Part model, mm, in its own coordinate system. Face numbers are marked on the shaded views. A direction names the side the tool comes from. Give positions to 0.01 mm unless a question says otherwise; leave off trailing zeros. Order: outer loops, then holes, each group sorted by start corner. A loop starts at its lowest first (then second) coordinate and runs counter-clockwise, first axis right, second up. Notation, with made-up numbers: (63, 76.25) - (95, 76.25) arc R30 cw to (95, 99.25) - close; hole circle Ø11 at (-33.5, -25.75). An arc over 180 degrees is marked (long way). One line per item, written item: value.
```python
from build123d import *

# Parameters (mm, degrees)
BOSS_EXTRU_1_DEPTH      = 9
ESQUISSE2_R             = 1
ENL_V_MAT_EXTRU_1_DEPTH = 16.588457268


with BuildPart() as part:
    # Esquisse1 → Boss.-Extru.1 (new body)
    with BuildSketch(Plane(origin=(0, 0, 0), x_dir=(1, 0, 0), z_dir=(0, 1, 0))):
        with BuildLine():
            Line((3.968626967, 0.5), (8.986100378, 0.5))
            ThreePointArc((8.986100378, 0.5), (-9, 0), (8.986100378, -0.5))
            Line((8.986100378, -0.5), (3.968626967, -0.5))
            ThreePointArc((3.968626967, -0.5), (0, -4), (-3.968626967, -0.5))
            Line((-3.968626967, -0.5), (-5, -0.5))
            Line((-5, -0.5), (-5, 0.5))
            Line((-5, 0.5), (-3.968626967, 0.5))
            ThreePointArc((-3.968626967, 0.5), (0, 4), (3.968626967, 0.5))
        make_face()
    extrude(amount=BOSS_EXTRU_1_DEPTH)

    # Esquisse2 → Enlèv. mat.-Extru.1 (cut, through all)
    with BuildSketch(Plane(origin=(0, 9, 0), x_dir=(1, 0, 0), z_dir=(0, 1, 0))):
        with Locations(Location((0, -6.5, 0), (0, 0, 270))):
            Circle(ESQUISSE2_R)
        with Locations(Location((0, 6.5, 0), (0, 0, 270))):
            Circle(ESQUISSE2_R)
    extrude(amount=-ENL_V_MAT_EXTRU_1_DEPTH, mode=Mode.SUBTRACT)


solid = part.part
```
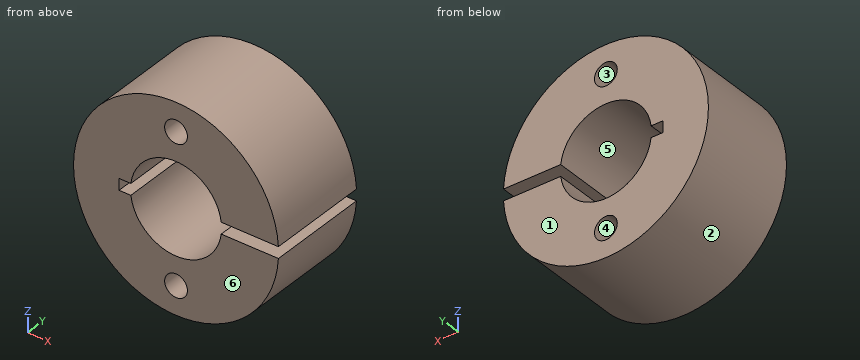
1) Cut at B-B, the plane x = 0. Give the cut face in (y, z), then the cut area to 3 significant figures.
Outcome:
outline: (0, -9) - (9, -9) - (9, -7.5) - (0, -7.5) - close; (0, -5.5) - (9, -5.5) - (9, -4) - (0, -4) - close; (0, 4) - (9, 4) - (9, 5.5) - (0, 5.5) - close; (0, 7.5) - (9, 7.5) - (9, 9) - (0, 9) - close
area: 54.0 mm^2
2) Cut at D-D, the plane x = -2.25. Give the cut face in (y, z).
Outcome:
outline: (0, -8.71) - (9, -8.71) - (9, -3.31) - (0, -3.31) - close; (0, 3.31) - (9, 3.31) - (9, 8.71) - (0, 8.71) - close
3) Drill centre lines: line 1 along X through (y, z) = (4.25, 6.5); line 2 along Z through (x, y) = (-0.25, 7.25); line 3 along Z through (x, y) = (-1.25, 7). Where is each one in solid material? Low to high. Write a range as from..to.
Outcome:
line 1: x = -6.22..-1, 1..6.22
line 2: z = -9..-7.47, -5.53..-3.99, 3.99..5.53, 7.47..9
line 3: z = -8.91..-3.8, 3.8..8.91
4) Which spindle directions (+Z, -Z, +X, -X, +Y, -Y) get a long thin tool onto all of the face, cutting with end or side? Do the marked faces 5 and 6. Say none if no direction does.
Outcome:
face 5: +Y, -Y
face 6: +Z, -Z, +X, -X, -Y
5) Mould opens along Z. For the marked faces 1, 2, 3 and 4 say: released by +Z, released by -Z, zero draft, split by the parting line, or undercut.
Outcome:
face 1: zero draft
face 2: split by the parting line
face 3: undercut
face 4: undercut
6) Cut at A-A, the plane y = 1.5. Give the cut face in (x, z), then the cut area to 3 significant figures.
Outcome:
outline: (-5, -0.5) - (-5, 0.5) - (-3.97, 0.5) arc R4 cw to (3.97, 0.5) - (8.99, 0.5) arc R9 ccw (long way) to (8.99, -0.5) - (3.97, -0.5) arc R4 cw to (-3.97, -0.5) - close; hole circle Ø2 at (0, -6.5); hole circle Ø2 at (0, 6.5)
area: 192 mm^2
7) Cut at C-C, the plane z = 3.25. Give the cut face in (x, y), then the cut area to 3 significant figures.
Outcome:
outline: (-8.39, 0) - (-2.33, 0) - (-2.33, 9) - (-8.39, 9) - close; (2.33, 0) - (8.39, 0) - (8.39, 9) - (2.33, 9) - close
area: 109 mm^2
8) Pin check, flat tips, straight feed: pin 1 (1.5 mm diameter, centred on x = 5, y = 6.5, fed in from -Z); pin 2 (1.2 mm diameter, centred on x = 0, z = -6.5, fed in from -Y); pin 3 (4 mm diameter, centred on x = 5.5, y = 2.5, fed in from +Z); pin 4 (3 mm diameter, centred on x = 0, z = 6.5, fed in from +Y). Stop position of each tip, or through.
Outcome:
pin 1: stops at z = -7.93
pin 2: passes through
pin 3: stops at z = 8.29
pin 4: stops at y = 9
